Source: CAD feature listing. Evaluate the final solid. Frame: model axes, mm. A direction names the side the tool comes from. Give positions to 0.01 mm unless a question says otherwise; leave off trailing zeros. Loops run counter-clockwise (first coordinate to the right, second up) from the corner with the lowest first, then second, coordinate; pieces in that order, holes last. Notation, with made-up numbers: M 69,-7 L 84,-7 A21 ccw 84,3 Z; hole C 32,-9.75 d1. An arc over 180 degrees is marked long. Answer in a Markdown table with one row per item.
```python
from build123d import *

# Parameters (mm, degrees)
SKETCH1_W           = 7
SKETCH1_H           = 7
BOSS_EXTRUDE1_DEPTH = 8
SKETCH2_W           = 3
SKETCH2_H           = 3
CUT_EXTRUDE1_DEPTH  = 9
CUT_EXTRUDE2_DEPTH  = 6
CUT_EXTRUDE3_DEPTH  = 6
SKETCH5_W           = 1
SKETCH5_H           = 2
CUT_EXTRUDE4_DEPTH  = 1
CUT_EXTRUDE5_DEPTH  = 4
SKETCH7_W           = 2
SKETCH7_H           = 3
CUT_EXTRUDE6_DEPTH  = 2
CUT_EXTRUDE7_DEPTH  = 6


with BuildPart() as part:
    # Sketch1 → Boss-Extrude1 (new body)
    with BuildSketch(Plane.XY):
        Rectangle(SKETCH1_W, SKETCH1_H)
    extrude(amount=BOSS_EXTRUDE1_DEPTH)

    # Sketch2 → Cut-Extrude1 (cut, through all)
    with BuildSketch(Plane.XY.offset(8)):
        with Locations((0, -2)):
            Rectangle(SKETCH2_W, SKETCH2_H)
    extrude(amount=-CUT_EXTRUDE1_DEPTH, mode=Mode.SUBTRACT)

    # Sketch3 → Cut-Extrude2 (cut)
    with BuildSketch(Plane(origin=(3.5, 0, 0), x_dir=(0, 0, -1), z_dir=(1, 0, 0))):
        Polygon((-8, -2.5), (-2, 3.5), (-8, 3.5), align=None)
    extrude(amount=-CUT_EXTRUDE2_DEPTH, mode=Mode.SUBTRACT)

    # Sketch4 → Cut-Extrude3 (cut)
    with BuildSketch(Plane(origin=(-2.5, 0, 0), x_dir=(0, 0, -1), z_dir=(1, 0, 0))):
        Polygon((-5, 3.5), (-5, 0.5), (-8, -2.5), (-8, 3.5), align=None)
    extrude(amount=-CUT_EXTRUDE3_DEPTH, mode=Mode.SUBTRACT)

    # Sketch5 → Cut-Extrude4 (cut)
    with BuildSketch(Plane(origin=(3.5, 0, 0), x_dir=(0, 0, -1), z_dir=(1, 0, 0))):
        with Locations((-7.5, -2.5)):
            Rectangle(SKETCH5_W, SKETCH5_H)
    extrude(amount=-CUT_EXTRUDE4_DEPTH, mode=Mode.SUBTRACT)

    # Sketch6 → Cut-Extrude5 (cut)
    with BuildSketch(Plane(origin=(3.5, 0, 0), x_dir=(0, 0, -1), z_dir=(1, 0, 0))):
        Polygon((0, 3.5), (-2, 3.5), (-5, 0.5), (-3, 0.5), (-1, 2.5), (0, 2.5), align=None)
    extrude(amount=-CUT_EXTRUDE5_DEPTH, mode=Mode.SUBTRACT)

    # Sketch7 → Cut-Extrude6 (cut)
    with BuildSketch(Plane(origin=(0, 2.5, 0), x_dir=(1, 0, 0), z_dir=(0, 1, 0))):
        with Locations((2.5, -1.5)):
            Rectangle(SKETCH7_W, SKETCH7_H)
    extrude(amount=-CUT_EXTRUDE6_DEPTH, mode=Mode.SUBTRACT)

    # Sketch8 → Cut-Extrude7 (cut)
    with BuildSketch(Plane(origin=(0, 0, 0), x_dir=(-1, 0, 0), z_dir=(0, 0, -1))):
        Polygon((-2.5, 0.5), (-3.5, -0.5), (-3.5, 0.5), align=None)
    extrude(amount=-CUT_EXTRUDE7_DEPTH, mode=Mode.SUBTRACT)


solid = part.part
```
Q1. Section query D-D (z = 3.5). Output: boundary loops of the cut face in (x, y), plus the area to 3 significant figures.
Values follow:
| item | result |
|---|---|
| outline | M -3.5,-3.5 L -1.5,-3.5 L -1.5,-0.5 L 1.5,-0.5 L 1.5,-3.5 L 3.5,-3.5 L 3.5,-0.5 L 2.5,0.5 L -0.5,0.5 L -0.5,2 L -2.5,2 L -2.5,3.5 L -3.5,3.5 Z |
| area | 24.5 mm^2 |
Q2. Section query B-B (z = 6.75). Output: boundary loops of the cut face in (x, y), plus the area to 3 significant figures.
Values follow:
| item | result |
|---|---|
| outline | M -3.5,-3.5 L -1.5,-3.5 L -1.5,-1.25 L -3.5,-1.25 Z; M 1.5,-3.5 L 3.5,-3.5 L 3.5,-1.25 L 1.5,-1.25 Z |
| area | 9.00 mm^2 |
Q3. Section query A-A (y = -2). Output: boundary loops of the cut face in (x, z).
Values follow:
| item | result |
|---|---|
| outline | M -3.5,0 L -1.5,0 L -1.5,7.5 L -3.5,7.5 Z; M 1.5,0 L 3.5,0 L 3.5,7 L 2.5,7 L 2.5,7.5 L 1.5,7.5 Z |
Q4. Contact query for flat-ended pins moving along their axis: pin 1 Ø0.9 at (y, z) = (2.5, 3) entering from +X; pin 2 Ø2.5 at (x, z) = (0, 4) entering from -Y; pin 3 Ø3 at (x, y) = (1, -1) entering from +Z. Output: stop coordinate, or through.
Values follow:
| item | result |
|---|---|
| pin 1 | x = -0.5 |
| pin 2 | y = -0.5 |
| pin 3 | z = 7.91 |
Q5. Mould query, pull axis X, two halves, no side actions, for faces 1 (the flat face through (1.5, -2, 4)), 2 (the flat face through (-1, 0, 0)), 3 (the flat face through (3.5, -2, 3)). Classes: +X half, -X half, draft (parallel to the pull), parting line (faces both ways), or undercut.
Values follow:
| item | result |
|---|---|
| face 1 | undercut |
| face 2 | draft |
| face 3 | +X half |
Q6. Section query C-C (y = 1). Output: boundary loops of the cut face in (x, z), plus the area to 3 significant figures.
Values follow:
| item | result |
|---|---|
| outline | M -3.5,0 L 1.5,0 L 1.5,2.5 L -0.5,2.5 L -0.5,4.5 L -2.5,4.5 L -2.5,5 L -3.5,5 Z |
| area | 19.0 mm^2 |
Q7. Reachability of faces 4 (the flat face through (-3, 2, 5)), 5 (the flat face through (-2.5, 2, 4)), 6 (the flat face through (0.5, 2.5, 0.5)) from +Z, -Z, +X, -X, +Y, -Y: full face, straight path, thin tool, end or side. Return the list, or none.
Values follow:
| item | result |
|---|---|
| face 4 | +Z, +X, -X, +Y |
| face 5 | +Z, +X, +Y |
| face 6 | +Z, -Z, +X, +Y |
Q8. Ray query, probe 1 along X at (y, z) = (-2.75, 1.75); probe 2 along Y at (x, z) = (0.25, 4.5); probe 3 along Y at (x, z) = (2.75, 5.5). Return the intervals inside material, ascending. Write a range as from..to.
Values follow:
| item | result |
|---|---|
| probe 1 | -3.5..-1.5, 1.5..3.5 |
| probe 2 | -0.5..0.5 |
| probe 3 | -3.5..0 |
